Autodesk Inventor part; units mm, degrees
ref_plane "YZ Plane" through (0, 0, 0) normal (1, 0, 0) x (0, 1, 0)
ref_plane "XZ Plane" through (0, 0, 0) normal (0, 1, 0) x (-1, 0, 0)
ref_plane "XY Plane" through (0, 0, 0) normal (0, 0, 1) x (1, 0, 0)
sketch "Sketch1" plane through (0, 0, 0) normal (0, 1, 0) x (-1, 0, 0)
  arc A0 (20, 9.3923) -> (-20, 9.3923) centre (0, 9.3923) ccw
  line L0 (-20, -15.6077) -> (20, -15.6077)
  line L1 (20, -15.6077) -> (20, 9.3923)
  line L2 (-20, 9.3923) -> (-20, -15.6077)
  point P0 (0, 0)
  dimension "d0" = 40
extrude "Extrusion1" add sketch "Sketch1" along normal blind 50
sketch "Sketch2" plane through (0, 50, 0) normal (0, 1, 0) x (1, 0, 0)
  arc A0 (-20, -9.3923) -> (20, -9.3923) centre (0, -9.3923) ccw
  circle A1 centre (0, -9.3923) radius 3.75
  point P0 (0, 0)
  dimension "d4" = 7.5
extrude "Extrusion2" add sketch "Sketch2" along normal blind 10
sketch "Sketch3" plane through (0, 60, 9.3923) normal (0, 1, 0) x (1, 0, 0)
  circle A0 centre (0, 0) radius 3.75
  ellipse E0 centre (0, 0) end of major axis (-13, -14) minor radius 3.6924 (-2.25, 3) -> (-3.1582, 2.0219) ccw
  ellipse E1 centre (0, 0) end of major axis (13, -14) minor radius 3.7302 (-3, -2.25) -> (-2.4658, -2.8253) ccw
  ellipse E2 centre (0, 0) end of major axis (-13, -14) minor radius 3.6924 (-4.9841, -0.0284) -> (-0.0262, -5.3386) ccw
  ellipse E3 centre (0, 0) end of major axis (-13, -14) minor radius 3.6924 (2.25, -3) -> (3.1582, -2.0219) ccw
  ellipse E4 centre (0, 0) end of major axis (-13, -14) minor radius 3.6924 (4.9841, 0.0284) -> (0.0262, 5.3386) ccw
  ellipse E5 centre (0, 0) end of major axis (13, -14) minor radius 3.7302 (-0.0262, -5.3386) -> (4.9841, 0.0284) ccw
  ellipse E6 centre (0, 0) end of major axis (13, -14) minor radius 3.7302 (3, 2.25) -> (2.4658, 2.8253) ccw
  ellipse E7 centre (0, 0) end of major axis (13, -14) minor radius 3.7302 (0.0262, 5.3386) -> (-4.9841, -0.0284) ccw
  line L0 (8, 9) -> (-8, -9) construction
  line L1 (-8, 9) -> (8, -9) construction
  circle A1 centre (-8, 9) radius 1.5
  circle A2 centre (8, 9) radius 1.5
  circle A3 centre (8, -9) radius 1.5
  circle A4 centre (-8, -9) radius 1.5
  point P0 (0, 9.3923)
  dimension "d7" = 3
  dimension "d8" = 3
  dimension "d9" = 3
  dimension "d10" = 3
extrude "Extrusion3" add sketch "Sketch3" along normal blind 2.5
sketch "Sketch4" plane through (0, 60, 9.3923) normal (0, 1, 0) x (1, 0, 0)
  circle A0 centre (0, 0) radius 3.75
  point P0 (0, 9.3923)
extrude "Extrusion4" add sketch "Sketch4" along normal blind 2.5
properties part number "servo" material "Aluminum 6061, Welded"
For this review, take the finished solid that the model builds, in its own axes (mm). A direction names the side the tool comes from. Give positions to 0.01 mm unless a question says otherwise; leave off trailing zeros. Loops run counter-clockwise (first coordinate to the right, second up) from the corner with the lowest first, then second, coordinate; pieces in that order, holes last. Notation, with made-up numbers: M 55.5,62.25 L 107.5,62.25 A33 ccw 107.5,90.25 Z; hole C 45,59 d11. An arc over 180 degrees is marked long. One line per item, written item: value. Start each with the question number.
Q1. Machinability: for faces 1 (the face through (0, 0, 7)), 2 (the face through (6.81, 61.23, -0.52)), which of the approach directions +Z, -Z, +X, -X, +Y, -Y give a long, thin tool a straight path to every point of the face, cutting with its end or side? Answer none if there is none.
Q2. Clearance check with flat-ended pins moving along their axes: pin 1 Ø10 at (x, y) = (15, 32.5) entering from +Z; pin 2 Ø10 at (y, z) = (15, 21.5) entering from -X; pin 3 Ø3 at (x, z) = (1.5, -4) entering from +Y. State where each tip first meets the part, or that it passes through.
Q3. Add section B-B (x = -7.5). Count the separate pieces of the cut face and the enclosed holes in it, and give its area (3 significant figures).
Q4. For L1, parallel to Z at x = 8, y = 61; L2, parallel to Y at x = -11, z = 20; L3, parallel to Y at x = 0, z = -11.5, list the stretches that pass through material, from the lowest coordinate up.
Q5. Draft analysis for pull direction X (two halves, no side actions). For faces 3 (the face through (-0.81, 54.93, 5.73)), 4 (the face through (0, 62.5, 9)), 5 (the face through (6.81, 61.23, 17.48)), state which applies: released by +X, released by -X, zero draft, split by the parting line, or undercut.
Q6. Add section D-D (x = 16). Give the boundary of the cut face in (y, z).
Q7. Add section A-A (y = 40.5). Give the boundary of the cut face in (x, z), and give its area (3 significant figures).
Reply:
1. face 1: +Z, -Z, +X, -X, -Y
1. face 2: +Y
2. pin 1: z = 26.71
2. pin 2: x = -18.69
2. pin 3: y = 50
3. separate pieces: 5
3. enclosed holes: 0
3. area: 2,210 mm²
4. L1: -2.8 to -1.11, 1.89 to 5.68, 13.05 to 16.89, 19.89 to 21.61
4. L2: 0 to 50, 60 to 62.5
4. L3: 0 to 50
5. face 3: split by the parting line
5. face 4: zero draft
5. face 5: undercut
6. outline: M 0,-15.61 L 50,-15.61 L 50,21.39 L 0,21.39 Z
7. outline: M -20,-15.61 L 20,-15.61 L 20,9.39 A20 ccw -20,9.39 Z
7. area: 1,630 mm²
